Geometry check sheet. Reference: drawing and pictorial views, mm from the part's lowest x, y, z. A direction names the side the tool comes from. Coordinates: 2 decimals unless noted, no trailing zeros. Loops run counter-clockwise (first coordinate to the right, second up) from the corner with the lowest first, then second, coordinate; pieces in that order, holes last. Notation, with made-up numbers: (50.5, -1.5) -> (66.5, -1.5) arc R26 ccw to (66.5, 16.5) -> close; hole circle Ø3 at (62, 36). An arc over 180 degrees is marked (long way). Use CSV: the item, a comma, the result in double quotes.
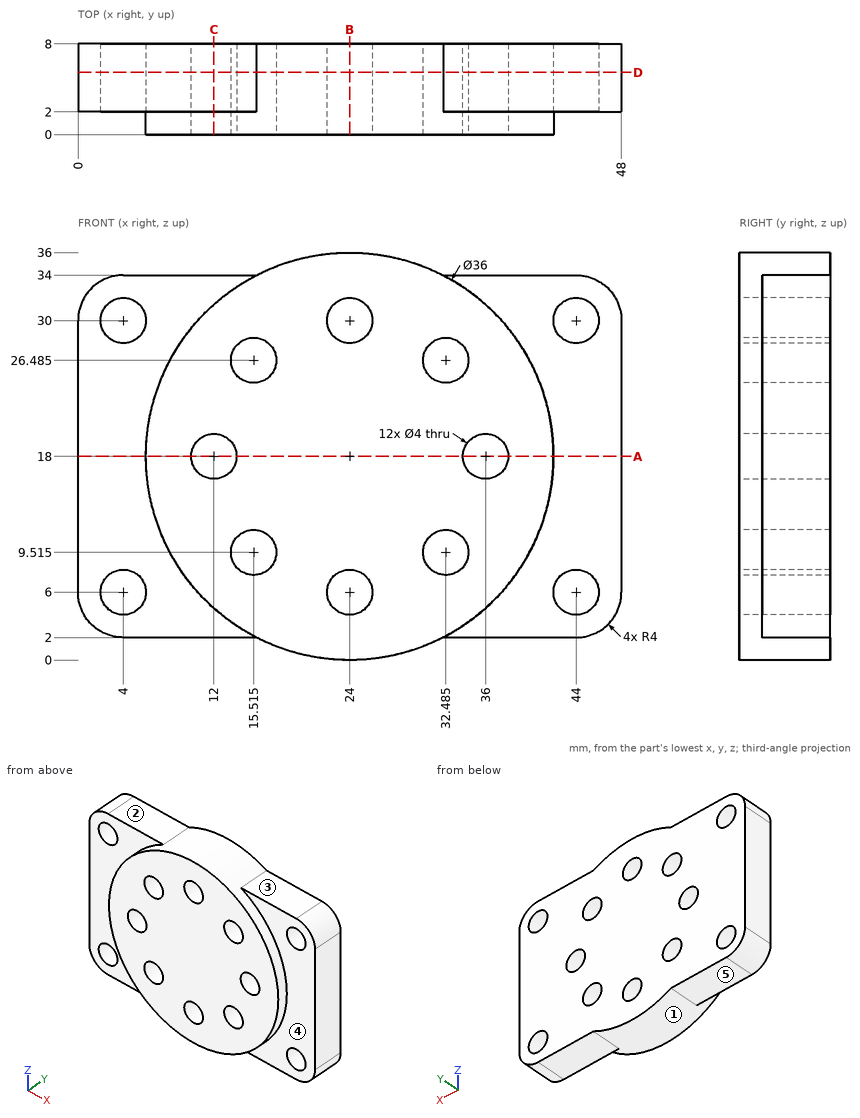
1) Cross-section at C-C on x = 12. Record the boundary of the cut face in (y, z).
Answer below:
outline,"(0, 4.58) -> (2, 4.58) -> (2, 2) -> (8, 2) -> (8, 16) -> (0, 16) -> close; (0, 20) -> (8, 20) -> (8, 34) -> (2, 34) -> (2, 31.42) -> (0, 31.42) -> close"
2) Go/stop test with flat-tipped pins: pin 1 Ø4 at (x, y) = (37.5, 1.5) entering from -Z; pin 2 Ø4.5 at (x, z) = (39.5, 24.5) entering from -Y; pin 3 Ø1.5 at (y, z) = (5.5, 31.5) entering from +X. Record where each tip stops, or that it passes through.
Answer below:
pin 1,"stops at z = 2"
pin 2,"stops at y = 0"
pin 3,"stops at x = 47.93"
3) Cross-section at A-A on z = 18. Record the boundary of the cut face in (x, y).
Answer below:
outline,"(0, 2) -> (6, 2) -> (6, 0) -> (10, 0) -> (10, 8) -> (0, 8) -> close; (14, 0) -> (34, 0) -> (34, 8) -> (14, 8) -> close; (38, 0) -> (42, 0) -> (42, 2) -> (48, 2) -> (48, 8) -> (38, 8) -> close"
4) Cross-section at B-B on x = 24. Record the boundary of the cut face in (y, z), and give its area (3 significant figures).
Answer below:
outline,"(0, 0) -> (8, 0) -> (8, 4) -> (0, 4) -> close; (0, 8) -> (8, 8) -> (8, 28) -> (0, 28) -> close; (0, 32) -> (8, 32) -> (8, 36) -> (0, 36) -> close"
area,"224 mm²"
5) Cross-section at D-D on y = 5.5. Give the number of separate pieces and of enclosed holes in the cut face, and give its area (3 significant figures).
Answer below:
separate pieces,"1"
enclosed holes,"12"
area,"1,420 mm²"
6) Thickness scan on line 1 along Z through (x, y) = (4, 5.95); line 2 along Z through (x, y) = (36, 2.25); line 3 along Z through (x, y) = (15, 3). Record the ranges inside material, lowest first. Write a range as from..to.
Answer below:
line 1,"z = 2..4, 8..28, 32..34"
line 2,"z = 2..16, 20..34"
line 3,"z = 2..7.58, 11.45..24.55, 28.42..34"
7) Access from +Z, -Z, +X, -X, +Y, -Y to the whole of each face (thin tool, end or side, straight path). Record for the marked faces 1, 2, 3, 4 and 5.
Answer below:
face 1,"-Y"
face 2,"+Z, -X, +Y, -Y"
face 3,"+Z, +X, +Y, -Y"
face 4,"+X, -Y"
face 5,"-Z, -X, +Y, -Y"
